Here's how the part is built. I have some questions about the finished solid (model axes, mm). A direction names the side the tool comes from. Round coordinates to 2 decimals unless told otherwise and drop trailing zeros. Write each loop counter-clockwise with the first axis right and the second up, starting at its lowest first coordinate (ties: lowest second). Pieces come first, ordered by that corner, then holes. Notation, with made-up numbers: (16, 1) -> (29, 1) arc R14 cw to (29, 25) -> close; hole circle Ø6 at (0, 44.5). An arc over 180 degrees is marked (long way). Answer as CSV lines item,"result".
```python
from build123d import *

# Parameters (mm, degrees)
SKETCH1_R                    = 1.5
SKETCH1_R_2                  = 2.7
BOSS_EXTRUDE1_DEPTH          = 7.5
SKETCH3_R                    = 8
CUT_EXTRUDE2_DEPTH           = 5
FILLET2_R                    = 20
TALADRO_DE_MARGEN_PARA_M41_D = 4.8
FILLET3_R                    = 5
CHAMFER1_SIZE                = 2.5
SKETCH7_W                    = 10.89
SKETCH7_H                    = 9.13
SKETCH7_W_2                  = 8.49
SKETCH7_H_2                  = 6.73
BOSS_EXTRUDE2_DEPTH          = 15
FILLET5_R                    = 2.5


with BuildPart() as part:
    # Sketch1 → Boss-Extrude1 (new body)
    with BuildSketch(Plane.XY):
        with BuildLine():
            Line((42.669600757, 14), (42.669600757, 21.1))
            Line((42.669600757, 21.1), (84.869600757, 21.1))
            Line((84.869600757, 21.1), (84.869600757, -21.1))
            Line((84.869600757, -21.1), (42.669600757, -21.1))
            Line((42.669600757, -21.1), (42.669600757, -14))
            Line((42.669600757, -14), (9.223174911, -25.907200632))
            ThreePointArc((9.223174911, -25.907200632), (-27.5, 0), (9.223174911, 25.907200632))
            Line((9.223174911, 25.907200632), (42.669600757, 14))
        make_face()
        with Locations((79.269600757, 15.5)):
            Circle(SKETCH1_R, mode=Mode.SUBTRACT)
        with Locations((79.269600757, -15.5)):
            Circle(SKETCH1_R, mode=Mode.SUBTRACT)
        Circle(SKETCH1_R_2, mode=Mode.SUBTRACT)
    extrude(amount=BOSS_EXTRUDE1_DEPTH)

    # Sketch3 → Cut-Extrude2 (cut)
    with BuildSketch(Plane.XY.offset(7.5)):
        Circle(SKETCH3_R)
    extrude(amount=-CUT_EXTRUDE2_DEPTH, mode=Mode.SUBTRACT)

    # Fillet2
    # the kernel refuses this fillet: 20 mm, written as the material it adds along each edge
    with BuildSketch(Plane(origin=(42.669600757, -14, 0), x_dir=(-0.9420800229659998, -0.3353881785757827, 0), z_dir=(0, 0, 1))) as fillet2_piece_1:
        with BuildLine():
            CenterArc((17.308114645, 20), FILLET2_R, 221.725423621, 48.274576379)
            Line((2.381256068, 6.688768163), (2.082718896, 6.422543526))
            ThreePointArc((2.082718896, 6.422543526), (0.813796025, 3.478539353), (-0.376832009, 0.134155271))
            Line((-0.376832009, 0.134155271), (0, -0.4))
            Line((0, -0.4), (17.308114645, -0.4))
            Line((17.308114645, -0.4), (17.308114645, 0))
        make_face()
    extrude(amount=7.5)
    with BuildSketch(Plane(origin=(42.669600757, 14, 0), x_dir=(-0.9420800229659999, 0.3353881785757825, 0), z_dir=(0, 0, 1))) as fillet2_piece_2:
        with BuildLine():
            CenterArc((17.308114645, -20), FILLET2_R, 90, 48.274576379)
            Line((2.381256068, -6.688768163), (2.082718896, -6.422543526))
            ThreePointArc((2.082718896, -6.422543526), (0.813796025, -3.478539353), (-0.376832009, -0.134155271))
            Line((-0.376832009, -0.134155271), (0, 0.4))
            Line((0, 0.4), (17.308114645, 0.4))
            Line((17.308114645, 0.4), (17.308114645, 0))
        make_face()
    extrude(amount=7.5)

    # Taladro de margen para M41 (through all)
    with Locations(Plane.XY.offset(7.5)):
        with Locations((79.269600757, -15.5), (79.269600757, 15.5)):
            Hole(TALADRO_DE_MARGEN_PARA_M41_D / 2)

    # Fillet3
    fillet3_edges = [part.edges().sort_by_distance(p)[0] for p in [
        (42.669600757, 21.1, 3.75),
        (84.869600757, 21.1, 3.75),
        (84.869600757, -21.1, 3.75),
        (42.669600757, -21.1, 3.75),
    ]]
    fillet(fillet3_edges, radius=FILLET3_R)

    # Chamfer1
    chamfer1_edges = [part.edges().sort_by_distance(p)[0] for p in [
        (17.793573313, -22.856068838, 0),
        (-27.5, 0, 0),
        (17.793573313, 22.856068838, 0),
        (34.118456698, 18.673946929, 0),
        (84.869600757, 0, 0),
        (61.870983905, 21.1, 0),
        (61.870983905, -21.1, 0),
        (34.118456698, -18.673946929, 0),
        (42.76478805, 20.975783912, 0),
        (42.76478805, -20.975783912, 0),
        (83.405134663, 19.635533906, 0),
        (83.405134663, -19.635533906, 0),
    ]]
    chamfer(chamfer1_edges, length=CHAMFER1_SIZE)

    # Sketch7 → Boss-Extrude2 (add)
    with BuildSketch(Plane(origin=(0, 0, 0), x_dir=(-1, 0, 0), z_dir=(0, 0, -1))):
        Rectangle(SKETCH7_W, SKETCH7_H)
        Rectangle(SKETCH7_W_2, SKETCH7_H_2, mode=Mode.SUBTRACT)
    extrude(amount=BOSS_EXTRUDE2_DEPTH)

    # Fillet5
    fillet5_edges = [part.edges().sort_by_distance(p)[0] for p in [
        (5.445, 4.565, -7.5),
        (5.445, -4.565, -7.5),
        (-5.445, -4.565, -7.5),
        (-5.445, 4.565, -7.5),
    ]]
    fillet(fillet5_edges, radius=FILLET5_R)


solid = part.part
```
1. Suppose I cut it at D-D on x = 17. Please give me the cut outline in (y, z), and give its area (3 significant figures).
Numbers:
outline,"(-23.14, 2.5) -> (-20.48, 0) -> (20.48, 0) -> (23.14, 2.5) -> (23.14, 7.5) -> (-23.14, 7.5) -> close"
area,"340 mm^2"
2. For pin 1 Ø3.5 at (y, z) = (1.5, -5) entering from +X (3 decimals); pin 2 Ø6 at (x, y) = (0, 0) entering from -Z; pin 3 Ø5.5 at (y, z) = (1, -7) entering from -X (3 decimals); pin 4 Ø4.5 at (x, y) = (79.27, -15.5) entering from +Z, each with a flat end and sliding along its axis, tell me the tip position at first contact or that it passes through.
Numbers:
pin 1,"stops at x = 5.445"
pin 2,"stops at z = 0"
pin 3,"stops at x = -5.445"
pin 4,"passes through"
3. If I drill on line 1 (Y direction, x = 0, z = 5.5); line 2 (Z direction, x = 5, y = 1); line 3 (Y direction, x = -1, z = -10.5) (3 decimals), over which ranges is the centre line in solid material (lowest first)?
Numbers:
line 1,"y = -27.5 to -8, 8 to 27.5"
line 2,"z = -15 to 2.5"
line 3,"y = -4.565 to -3.365, 3.365 to 4.565"
4. On a 3-axis mill with a long thin cutter (end or side, diameter ignored), from which of +Z, -Z, +X, -X, +Y, -Y can I reach the whole of each face in a straight line? I mean faces 4 (the face through (62.1, -19.9, 1.3)), 5 (the face through (0, -4.565, -7)), 6 (the face through (17.5, -21.652, 1.267)). Say none if no direction works.
Numbers:
face 4,"-Z, +X, -Y"
face 5,"-Z, +X, -X, -Y"
face 6,"-Z, -Y"
5. Suppose I cut it at A-A on x = 0. Please give me the cut outline in (y, z) (3 decimals), and give its area (3 significant figures).
Numbers:
outline,"(-27.5, 2.5) -> (-25, 0) -> (-4.565, 0) -> (-4.565, -15) -> (-3.365, -15) -> (-3.365, 0) -> (-2.7, 0) -> (-2.7, 2.5) -> (-8, 2.5) -> (-8, 7.5) -> (-27.5, 7.5) -> close; (2.7, 0) -> (3.365, 0) -> (3.365, -15) -> (4.565, -15) -> (4.565, 0) -> (25, 0) -> (27.5, 2.5) -> (27.5, 7.5) -> (8, 7.5) -> (8, 2.5) -> (2.7, 2.5) -> close"
area,"349 mm^2"
6. Suppose I cut it at B-B on z = -9.25. Please give me the cut outline in (x, y) (3 decimals).
Numbers:
outline,"(-5.445, -2.065) arc R2.5 ccw to (-2.945, -4.565) -> (2.945, -4.565) arc R2.5 ccw to (5.445, -2.065) -> (5.445, 2.065) arc R2.5 ccw to (2.945, 4.565) -> (-2.945, 4.565) arc R2.5 ccw to (-5.445, 2.065) -> close; hole (-4.245, -3.365) -> (4.245, -3.365) -> (4.245, 3.365) -> (-4.245, 3.365) -> close"
7. Suppose I cut it at C-C on x = 69.5. Please give me the cut outline in (y, z).
Numbers:
outline,"(-21.1, 2.5) -> (-18.6, 0) -> (18.6, 0) -> (21.1, 2.5) -> (21.1, 7.5) -> (-21.1, 7.5) -> close"
8. If we mould it in two halves opening along X, with no side actions, what happens to faces 1 (the face through (30, -1, 7.5)), 2 (the face through (83, 20, 5)), 3 (the face through (4.245, 0, -7))? For each: released by +X, released by -X, zero draft, split by the parting line, or undercut.
Numbers:
face 1,"zero draft"
face 2,"released by +X"
face 3,"undercut"
